Source: CAD feature listing. Evaluate the final solid. Frame: model axes, mm. Face numbers are marked on the shaded views. A direction names the side the tool comes from. Round coordinates to 2 decimals unless told otherwise and drop trailing zeros. Order: outer loops, then holes, each group sorted by start corner. A loop starts at its lowest first (then second) coordinate and runs counter-clockwise, first axis right, second up.
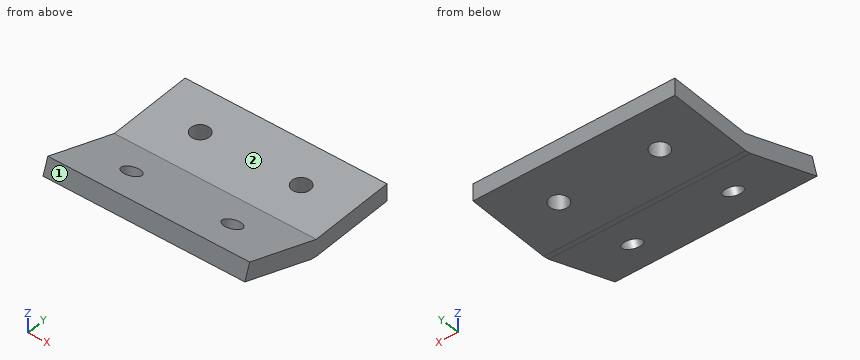
```python
from build123d import *

# Parameters (mm, degrees)
F1_DEPTH = 3
F3_DEPTH = 35
F5_DEPTH = 25


with BuildPart() as f1:
    # F0 (on Top) → F1 (new body)
    with BuildSketch(Plane.XY):
        with BuildLine():
            Line((-17.5, 0), (-17.5, -7.5))
            Line((-17.5, -7.5), (17.5, -7.5))
            Line((17.5, -7.5), (17.5, 0))
            Line((17.5, 0), (10.35, 0))
            ThreePointArc((10.35, 0), (8.75, -1.6), (7.15, 0))
            Line((7.15, 0), (0, 0))
            Line((0, 0), (-7.15, 0))
            ThreePointArc((-7.15, 0), (-8.75, -1.6), (-10.35, 0))
            Line((-10.35, 0), (-17.5, 0))
        make_face()
        with BuildLine():
            Line((-17.5, 7.5), (-17.5, 0))
            Line((-17.5, 0), (-10.35, 0))
            ThreePointArc((-10.35, 0), (-8.75, 1.6), (-7.15, 0))
            Line((-7.15, 0), (0, 0))
            Line((0, 0), (7.15, 0))
            ThreePointArc((7.15, 0), (8.75, 1.6), (10.35, 0))
            Line((10.35, 0), (17.5, 0))
            Line((17.5, 0), (17.5, 7.5))
            Line((17.5, 7.5), (-17.5, 7.5))
        make_face()
    extrude(amount=F1_DEPTH)

    # F2 (on face) → F3 (join)
    with BuildSketch(Plane.YZ.offset(17.5)):
        Polygon((-8.52606043, 0.1809221376), (-7.5, 3), (-21.5953893118, 8.1303021499), (-22.6214497418, 5.3112242875), align=None)
        Polygon((-7.5, 0), (-7.5, 3), (-8.52606043, 0.1809221376), align=None)
    extrude(amount=-F3_DEPTH)

    # F4 (on face) → F5 (cut)
    with BuildSketch(Plane(origin=(0, -0.9392123538, -2.580464734), x_dir=(1, 0, 0), z_dir=(0, -0.3420201433, -0.9396926208))):
        with BuildLine():
            Line((10.35, 15.5737550859), (7.15, 15.5737550859))
            ThreePointArc((7.15, 15.5737550859), (8.75, 13.9737550859), (10.35, 15.5737550859))
        make_face()
        with BuildLine():
            ThreePointArc((10.35, 15.5737550859), (8.75, 17.1737550859), (7.15, 15.5737550859))
            Line((7.15, 15.5737550859), (10.35, 15.5737550859))
        make_face()
        with BuildLine():
            Line((-10.35, 15.5737550859), (-7.15, 15.5737550859))
            ThreePointArc((-7.15, 15.5737550859), (-8.75, 17.1737550859), (-10.35, 15.5737550859))
        make_face()
        with BuildLine():
            ThreePointArc((-10.35, 15.5737550859), (-8.75, 13.9737550859), (-7.15, 15.5737550859))
            Line((-7.15, 15.5737550859), (-10.35, 15.5737550859))
        make_face()
    extrude(amount=-F5_DEPTH, mode=Mode.SUBTRACT)


solid = f1.part
```
1. Section B-B on x = 8.75. Return loops of the section in (y, z), plus the area to 3 significant figures.
2. Section D-D on y = -6.5. Return loops of the section in (x, z), plus the area to 3 significant figures.
3. First-contact query: pin 1 (2.5 mm diameter, centred on x = 8.75, y = 0, fed in from -Z); pin 2 (12 mm diameter, centred on x = -11, y = 3.5, fed in from +Z); pin 3 (1.5 mm diameter, centred on x = -12, y = -16, fed in from -Z). Flat tips, straight axial feed; report the tip coordinate or a pass-through.
4. Section A-A on y = 0. Return loops of the section in (x, z), plus the area to 3 significant figures.
5. Section C-C on x = -12.5. Return loops of the section in (y, z).
6. Line query: line 1 along X through (y, z) = (-0.5, 1); line 2 along Z through (x, y) = (0, 4.5); line 3 along Y through (x, z) = (-8.75, 2.45). Output: solid intervals per line, ascending.
7. Access query for the marked faces 1 and 2. Directions: +Z, -Z, +X, -X, +Y, -Y. A direction counts if a zero-diameter tool reaches every point of the face in a straight line with its end or side. Return the directions, or none.
Result:
1. outline: (-22.62, 5.31) - (-17.08, 3.29) - (-16.05, 6.11) - (-21.6, 8.13) - close; (-14.07, 2.2) - (-8.53, 0.18) - (-7.5, 0) - (-1.6, 0) - (-1.6, 3) - (-7.5, 3) - (-13.04, 5.02) - close; (1.6, 0) - (7.5, 0) - (7.5, 3) - (1.6, 3) - close
1. area: 72.3 mm2
2. outline: (-17.5, 0) - (17.5, 0) - (17.5, 3) - (-17.5, 3) - close
2. area: 105 mm2
3. pin 1: passes through
3. pin 2: stops at z = 3
3. pin 3: stops at z = 2.63
4. outline: (-17.5, 0) - (-10.35, 0) - (-10.35, 3) - (-17.5, 3) - close; (-7.15, 0) - (7.15, 0) - (7.15, 3) - (-7.15, 3) - close; (10.35, 0) - (17.5, 0) - (17.5, 3) - (10.35, 3) - close
4. area: 85.8 mm2
5. outline: (-22.62, 5.31) - (-8.53, 0.18) - (-7.5, 0) - (7.5, 0) - (7.5, 3) - (-7.5, 3) - (-21.6, 8.13) - close
6. line 1: x = -17.5 to -10.27, -7.23 to 7.23, 10.27 to 17.5
6. line 2: z = 0 to 3
6. line 3: y = -13.98 to -1.6, 1.6 to 7.5
7. face 1: +Z, +X, -X, -Y
7. face 2: +Z, +X, -X, +Y
